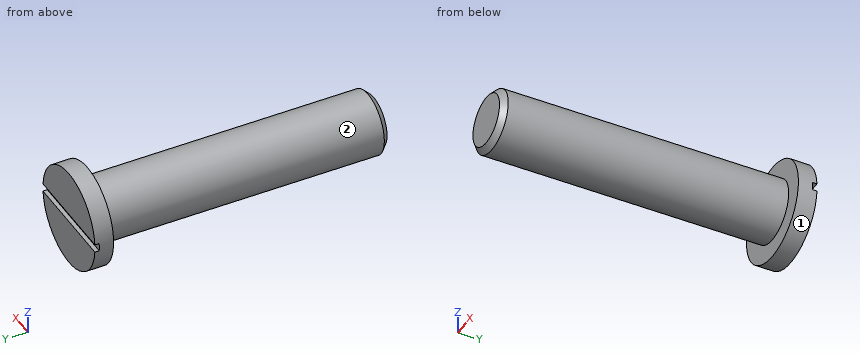
Autodesk Inventor part; units mm, degrees
ref_plane "hebel_XY" through (0, 24.5, 0) normal (0, 1, 0) x (-1, 0, 0)
ref_plane "hebel_YZ" through (0, 24.5, 0) normal (-1, 0, 0) x (0, 0, 1)
ref_plane "hebel_ZX" through (0, 24.5, 0) normal (0, 0, 1) x (0, 1, 0)
sketch "Skizze_1" plane through (0, 21.5, 0) normal (0, 1, 0) x (1, 0, 0)
  circle A0 centre (0, 0) radius 8
extrude "Extrusion1" add sketch "Skizze_1" along normal blind 3
sketch "Skizze_3" plane through (0, 0, 0) normal (0, 0, 1) x (1, 0, 0)
  line L0 (-8, 24.5) -> (-8, 23.8)
  line L1 (-8, 23.8) -> (8, 23.8)
  line L2 (8, 23.8) -> (8, 24.5)
  line L3 (8, 24.5) -> (-8, 24.5)
extrude "Extrusion2" cut sketch "Skizze_3" along normal mid plane 1.3
sketch "Skizze_2" plane through (0, 0, 0) normal (0, 0, 1) x (1, 0, 0)
  line L0 (0, -24.5) -> (0, 21.5)
  line L1 (0, 21.5) -> (5, 21.5)
  line L2 (5, 21.5) -> (5, -23.58)
  line L3 (5, -23.58) -> (4.08, -24.5)
  line L4 (4.08, -24.5) -> (0, -24.5)
  line L5 (0, -24.5) -> (0, 21.5)
revolve "Revolution1" add sketch "Skizze_2" angle 360 about axis through (0, -24.5, 0) along (0, -1, 0)
thread "Thread1"
ref_plane "hebel_XY" through (0, 24.5, 0) normal (0, 1, 0) x (-1, 0, 0)
ref_plane "hebel_YZ" through (0, 24.5, 0) normal (-1, 0, 0) x (0, 0, 1)
ref_plane "hebel_ZX" through (0, 24.5, 0) normal (0, 0, 1) x (0, 1, 0)
properties part number "May Tec 1.63.14041/3_Clamping stud 40x40"
Geometry check sheet. Reference: the model listing, model coordinates, mm. Face numbers are marked on the shaded views. A direction names the side the tool comes from. Give positions to 0.01 mm unless a question says otherwise; leave off trailing zeros. Loops run counter-clockwise (first coordinate to the right, second up) from the corner with the lowest first, then second, coordinate; pieces in that order, holes last. Notation, with made-up numbers: (43.25, -17.75) -> (73.25, -17.75) arc R32 ccw to (73.25, 19.25) -> close; hole circle Ø1 at (46, 31.5). An arc over 180 degrees is marked (long way). Answer in a Markdown table with one row per item. Add a question column.
1) Material ranges on probe 1 along Y at (x, z) = (-7, 2.25); probe 2 along Z at (x, y) = (0.75, 22); probe 3 along X at (y, z) = (9.5, -0.75), recorded low to high. Write a range as from..to.
2) Cross-section at A-A on z = 0. Record the boundary of the cut face in (x, y), and give its area (3 significant figures).
3) Cross-section at B-B on x = 0. Record the boundary of the cut face in (y, z).
4) Set-up check for the marked faces 1 and 2: record each of +Z, -Z, +X, -X, +Y, -Y from which the full face is reachable in a straight line by a thin tool's end or side.
5) Gauge pin test, flat ends, axial feed: P1, Ø8, axis at y = 7, z = -4.5, coming from the +X side; P2, Ø1, axis at x = -1.5, z = -0.5, coming from the +Y side; P3, Ø3, axis at y = -2, z = 5.5, coming from the +X side; P4, Ø2, axis at x = 2.5, y = 8.5, coming from the +Z side. Record the tip position at first contact, or that the pin passes through.
6) Cross-section at C-C on y = 19. Record the boundary of the cut face in (x, z), and give its area (3 significant figures).
Outcome:
| question | item | result |
|---|---|---|
| 1 | probe 1 | y = 21.5..24.5 |
| 1 | probe 2 | z = -7.96..7.96 |
| 1 | probe 3 | x = -4.94..4.94 |
| 2 | outline | (-8, 21.5) -> (-5, 21.5) -> (-5, -23.58) -> (-4.08, -24.5) -> (4.08, -24.5) -> (5, -23.58) -> (5, 21.5) -> (8, 21.5) -> (8, 23.8) -> (-8, 23.8) -> close |
| 2 | area | 496 mm^2 |
| 3 | outline | (-24.5, -4.08) -> (-23.58, -5) -> (21.5, -5) -> (21.5, -8) -> (24.5, -8) -> (24.5, -0.65) -> (23.8, -0.65) -> (23.8, 0.65) -> (24.5, 0.65) -> (24.5, 8) -> (21.5, 8) -> (21.5, 5) -> (-23.58, 5) -> (-24.5, 4.08) -> close |
| 4 | face 1 | +Y, -Y |
| 4 | face 2 | -Y |
| 5 | P1 | stops at x = 4.97 |
| 5 | P2 | stops at y = 24.5 |
| 5 | P3 | stops at x = 3 |
| 5 | P4 | stops at z = 4.77 |
| 6 | outline | circle Ø10 at (0, 0) |
| 6 | area | 78.5 mm^2 |
